Source: CAD feature listing. Evaluate the final solid. Frame: model axes, mm. Face numbers are marked on the shaded views. A direction names the side the tool comes from. Coordinates: 2 decimals unless noted, no trailing zeros. Order: outer loops, then holes, each group sorted by start corner. A loop starts at its lowest first (then second) coordinate and runs counter-clockwise, first axis right, second up. Notation, with made-up numbers: (59, 51.25) -> (110, 51.25) arc R12 ccw to (110, 66.25) -> close; hole circle Ø8 at (-14, 58.5). An arc over 180 degrees is marked (long way). Put each result on its own line as item: value.
from build123d import *

# Parameters (mm, degrees)
EXTRUDE_1_DEPTH     = 2
EXTRUDE_2_DEPTH     = 5
EXTRUDE_3_DEPTH     = 7
SKETCH_2_R          = 4
CUT_EXTRUDE_1_DEPTH = 9


with BuildPart() as part:
    # Sketch 1 → Extrude 1 (new body)
    with BuildSketch(Plane(origin=(0, 0, 0), x_dir=(1, 0, 0), z_dir=(0, 1, 0))):
        with BuildLine():
            ThreePointArc((7.666821131, 12.480029994), (19.416821131, 13.480029994), (31.166821131, 12.480029994))
            Line((31.166821131, 12.480029994), (31.166821131, 24.480029994))
            ThreePointArc((31.166821131, 24.480029994), (41.166821131, 34.480029994), (51.166821131, 24.480029994))
            Line((51.166821131, 24.480029994), (51.166821131, 12.480029994))
            Line((51.166821131, 12.480029994), (51.166821131, -5.519970006))
            ThreePointArc((51.166821131, -5.519970006), (48.237888943, -12.591037818), (41.166821131, -15.519970006))
            Line((41.166821131, -15.519970006), (-2.333178869, -15.519970006))
            ThreePointArc((-2.333178869, -15.519970006), (-9.404246681, -12.591037818), (-12.333178869, -5.519970006))
            Line((-12.333178869, -5.519970006), (-12.333178869, 12.480029994))
            Line((-12.333178869, 12.480029994), (-12.333178869, 24.480029994))
            ThreePointArc((-12.333178869, 24.480029994), (-2.333178869, 34.480029994), (7.666821131, 24.480029994))
            Line((7.666821131, 24.480029994), (7.666821131, 12.480029994))
        make_face()
    extrude(amount=EXTRUDE_1_DEPTH)

    # Sketch 1_3 → Extrude 2 (add)
    with BuildSketch(Plane(origin=(0, 0, 0), x_dir=(1, 0, 0), z_dir=(0, 1, 0))):
        with BuildLine():
            Line((30.166821131, 24.480029994), (30.166821131, 13.655987129))
            ThreePointArc((30.166821131, 13.655987129), (19.416821131, 14.480029994), (8.666821131, 13.655987129))
            Line((8.666821131, 13.655987129), (8.666821131, 24.480029994))
            ThreePointArc((8.666821131, 24.480029994), (-2.333178869, 35.480029994), (-13.333178869, 24.480029994))
            Line((-13.333178869, 24.480029994), (-13.333178869, 12.480029994))
            Line((-13.333178869, 12.480029994), (-13.333178869, -5.519970006))
            ThreePointArc((-13.333178869, -5.519970006), (-10.111353462, -13.298144599), (-2.333178869, -16.519970006))
            Line((-2.333178869, -16.519970006), (41.166821131, -16.519970006))
            ThreePointArc((41.166821131, -16.519970006), (48.944995724, -13.298144599), (52.166821131, -5.519970006))
            Line((52.166821131, -5.519970006), (52.166821131, 12.480029994))
            Line((52.166821131, 12.480029994), (52.166821131, 24.480029994))
            ThreePointArc((52.166821131, 24.480029994), (41.166821131, 35.480029994), (30.166821131, 24.480029994))
        make_face()
        with BuildLine():
            Line((-12.333178869, 12.480029994), (-12.333178869, 24.480029994))
            ThreePointArc((-12.333178869, 24.480029994), (-2.333178869, 34.480029994), (7.666821131, 24.480029994))
            Line((7.666821131, 24.480029994), (7.666821131, 12.480029994))
            ThreePointArc((7.666821131, 12.480029994), (19.416821131, 13.480029994), (31.166821131, 12.480029994))
            Line((31.166821131, 12.480029994), (31.166821131, 24.480029994))
            ThreePointArc((31.166821131, 24.480029994), (41.166821131, 34.480029994), (51.166821131, 24.480029994))
            Line((51.166821131, 24.480029994), (51.166821131, 12.480029994))
            Line((51.166821131, 12.480029994), (51.166821131, -5.519970006))
            ThreePointArc((51.166821131, -5.519970006), (48.237888943, -12.591037818), (41.166821131, -15.519970006))
            Line((41.166821131, -15.519970006), (-2.333178869, -15.519970006))
            ThreePointArc((-2.333178869, -15.519970006), (-9.404246681, -12.591037818), (-12.333178869, -5.519970006))
            Line((-12.333178869, -5.519970006), (-12.333178869, 12.480029994))
        make_face(mode=Mode.SUBTRACT)
    extrude(amount=EXTRUDE_2_DEPTH)

    # Sketch 1_4 → Extrude 3 (add)
    with BuildSketch(Plane(origin=(0, 0, 0), x_dir=(1, 0, 0), z_dir=(0, 1, 0))):
        with BuildLine():
            Line((-2.333178869, -17.519970006), (41.166821131, -17.519970006))
            ThreePointArc((41.166821131, -17.519970006), (49.652102505, -14.00525138), (53.166821131, -5.519970006))
            Line((53.166821131, -5.519970006), (53.166821131, 12.480029994))
            Line((53.166821131, 12.480029994), (53.166821131, 24.480029994))
            ThreePointArc((53.166821131, 24.480029994), (41.166821131, 36.480029994), (29.166821131, 24.480029994))
            Line((29.166821131, 24.480029994), (29.166821131, 14.81243236))
            ThreePointArc((29.166821131, 14.81243236), (19.416821131, 15.480029994), (9.666821131, 14.81243236))
            Line((9.666821131, 14.81243236), (9.666821131, 24.480029994))
            ThreePointArc((9.666821131, 24.480029994), (-2.333178869, 36.480029994), (-14.333178869, 24.480029994))
            Line((-14.333178869, 24.480029994), (-14.333178869, 12.480029994))
            Line((-14.333178869, 12.480029994), (-14.333178869, -5.519970006))
            ThreePointArc((-14.333178869, -5.519970006), (-10.818460243, -14.00525138), (-2.333178869, -17.519970006))
        make_face()
        with BuildLine():
            Line((30.166821131, 24.480029994), (30.166821131, 13.655987129))
            ThreePointArc((30.166821131, 13.655987129), (19.416821131, 14.480029994), (8.666821131, 13.655987129))
            Line((8.666821131, 13.655987129), (8.666821131, 24.480029994))
            ThreePointArc((8.666821131, 24.480029994), (-2.333178869, 35.480029994), (-13.333178869, 24.480029994))
            Line((-13.333178869, 24.480029994), (-13.333178869, 12.480029994))
            Line((-13.333178869, 12.480029994), (-13.333178869, -5.519970006))
            ThreePointArc((-13.333178869, -5.519970006), (-10.111353462, -13.298144599), (-2.333178869, -16.519970006))
            Line((-2.333178869, -16.519970006), (41.166821131, -16.519970006))
            ThreePointArc((41.166821131, -16.519970006), (48.944995724, -13.298144599), (52.166821131, -5.519970006))
            Line((52.166821131, -5.519970006), (52.166821131, 12.480029994))
            Line((52.166821131, 12.480029994), (52.166821131, 24.480029994))
            ThreePointArc((52.166821131, 24.480029994), (41.166821131, 35.480029994), (30.166821131, 24.480029994))
        make_face(mode=Mode.SUBTRACT)
    extrude(amount=EXTRUDE_3_DEPTH)

    # Sketch 2 → Cut-Extrude 1 (cut)
    with BuildSketch(Plane.XZ):
        with Locations((0.166821131, 0.519970006)):
            Circle(SKETCH_2_R)
        with Locations((40.166821131, 0.519970006)):
            Circle(SKETCH_2_R)
        Polygon((19.166821131, 0.519970006), (18.166821131, 0.519970006), (19.166821131, 1.519970006), (20.166821131, 0.519970006), align=None)
        with BuildLine():
            ThreePointArc((24.416821131, 9.519970006), (19.416821131, 11.519970006), (14.416821131, 9.519970006))
            ThreePointArc((14.416821131, 9.519970006), (13.709924579, 9.537211385), (13.727165958, 10.244107937))
            ThreePointArc((13.727165958, 10.244107937), (19.416821131, 12.519970006), (25.106476303, 10.244107937))
            ThreePointArc((25.106476303, 10.244107937), (25.123717683, 9.537211385), (24.416821131, 9.519970006))
        make_face()
    extrude(amount=-CUT_EXTRUDE_1_DEPTH, mode=Mode.SUBTRACT)


solid = part.part
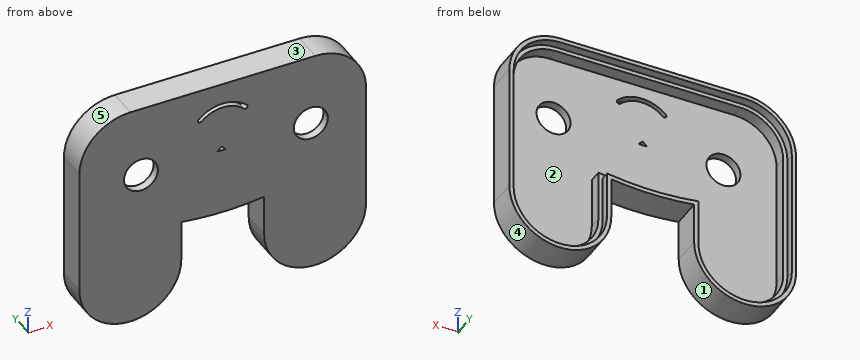
1. Cut plane D-D on z = -11. Output: boundary loops of the cut face in (x, y), plus the area to 3 significant figures.
Numbers:
outline: (-14.33, 0) -> (53.17, 0) -> (53.17, 7) -> (52.17, 7) -> (52.17, 5) -> (51.17, 5) -> (51.17, 2) -> (-12.33, 2) -> (-12.33, 5) -> (-13.33, 5) -> (-13.33, 7) -> (-14.33, 7) -> close
area: 151 mm2
2. First-contact query: pin 1 (3 mm diameter, centred on x = 45.5, z = -24, fed in from +Y); pin 2 (0.9 mm diameter, centred on x = 10.5, y = 4, fed in from -Z); pin 3 (1.5 mm diameter, centred on x = -1, y = 4.5, fed in from -Z); pin 4 (5 mm diameter, centred on x = 40.17, z = 0.52, fed in from +Y). Flat tips, straight axial feed; report the tip coordinate or a pass-through.
Numbers:
pin 1: stops at y = 2
pin 2: stops at z = -14.98
pin 3: stops at z = -36.47
pin 4: passes through
3. Cut plane C-C on x = 3. Output: boundary loops of the cut face in (y, z), plus the area to 3 significant figures.
Numbers:
outline: (0, -35.23) -> (7, -35.23) -> (7, -34.1) -> (5, -34.1) -> (5, -32.94) -> (2, -32.94) -> (2, -2.3) -> (0, -2.3) -> close; (0, 3.34) -> (2, 3.34) -> (2, 15.52) -> (5, 15.52) -> (5, 16.52) -> (7, 16.52) -> (7, 17.52) -> (0, 17.52) -> close
area: 111 mm2
4. Ray query, line 1 along X through (y, z) = (3.75, -16); line 2 along X through (y, z) = (4.5, -8.5); line 3 along X through (y, z) = (0.75, -20.5). Return the intervals inside material, ascending.
Numbers:
line 1: x = -14.33 to -12.33, 7.67 to 9.67, 29.17 to 31.17, 51.17 to 53.17
line 2: x = -14.33 to -12.33, 51.17 to 53.17
line 3: x = -14.33 to 9.67, 29.17 to 53.17
5. Cut plane B-B on y = 5.75. Output: boundary loops of the cut face in (x, z), plus the area to 3 significant figures.
Numbers:
outline: (-14.33, -24.48) arc R12 ccw to (9.67, -24.48) -> (9.67, -14.81) arc R71.53 ccw to (29.17, -14.81) -> (29.17, -24.48) arc R12 ccw to (53.17, -24.48) -> (53.17, 5.52) arc R12 ccw to (41.17, 17.52) -> (-2.33, 17.52) arc R12 ccw to (-14.33, 5.52) -> close; hole (-13.33, -24.48) arc R11 ccw to (8.67, -24.48) -> (8.67, -13.66) arc R70.53 ccw to (30.17, -13.66) -> (30.17, -24.48) arc R11 ccw to (52.17, -24.48) -> (52.17, 5.52) arc R11 ccw to (41.17, 16.52) -> (-2.33, 16.52) arc R11 ccw to (-13.33, 5.52) -> close
area: 253 mm2
6. Cut plane A-A on z = -21.5. Output: boundary loops of the cut face in (x, y), plus the area to 3 significant figures.
Numbers:
outline: (-14.33, 0) -> (9.67, 0) -> (9.67, 7) -> (8.67, 7) -> (8.67, 5) -> (7.67, 5) -> (7.67, 2) -> (-12.33, 2) -> (-12.33, 5) -> (-13.33, 5) -> (-13.33, 7) -> (-14.33, 7) -> close; (29.17, 0) -> (53.17, 0) -> (53.17, 7) -> (52.17, 7) -> (52.17, 5) -> (51.17, 5) -> (51.17, 2) -> (31.17, 2) -> (31.17, 5) -> (30.17, 5) -> (30.17, 7) -> (29.17, 7) -> close
area: 128 mm2
7. Pull-direction query (X, two-part tool) for the marked faces 3, 4 and 5; classes: pulls with the +X half, pulls with the -X half, needs draft (parallel to the pull), parting line crosses it, or undercut.
Numbers:
face 3: needs draft
face 4: undercut
face 5: pulls with the -X half
8. Set-up query: the marked faces 1 and 2. Return all of +Z, -Z, +X, -X, +Y, -Y with unobstructed straight access to the full face (end or side cutting, diameter ignored); none if empty.
Numbers:
face 1: -Z, +Y, -Y
face 2: +Y
